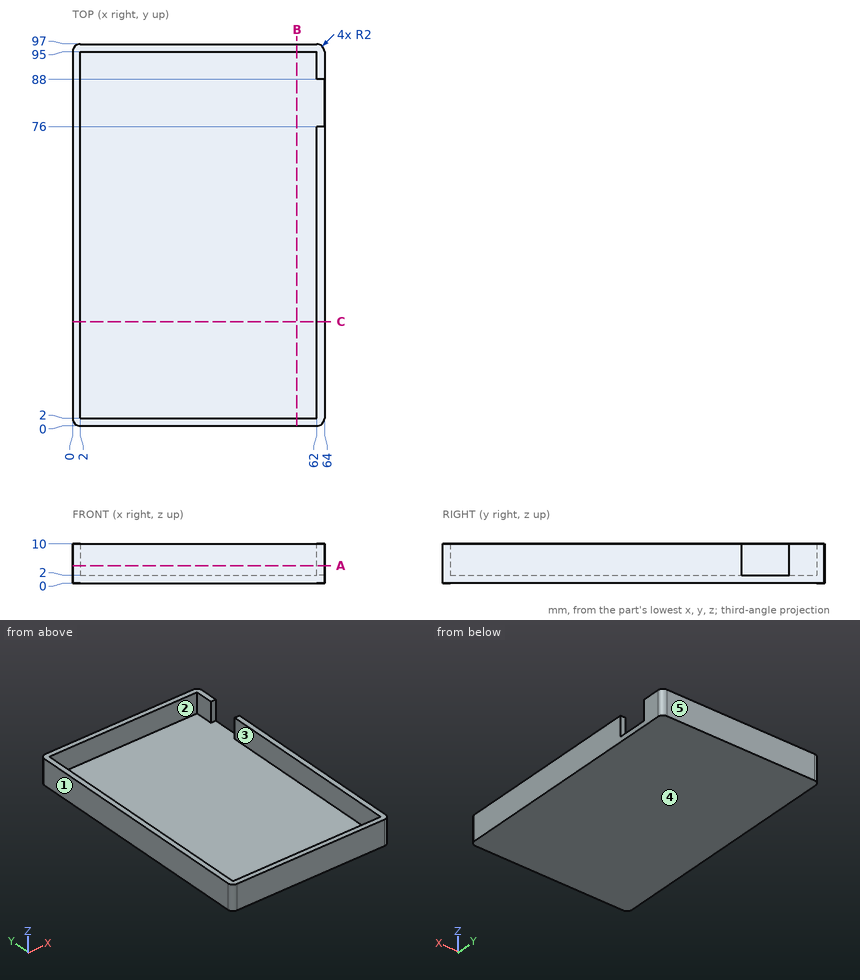
Input: dimensioned drawing with shaded views. Units: mm. Origin: part minimum x, y, z. A direction names the side the tool comes from. Give positions to 0.01 mm unless a question says otherwise; leave off trailing zeros. Order: outer loops, then holes, each group sorted by start corner. A loop starts at its lowest first (then second) coordinate and runs counter-clockwise, first axis right, second up. Notation, with made-up numbers: (56, 55) -> (78, 55) arc R16 cw to (78, 65) -> close; hole circle Ø6 at (42.5, 61). An arc over 180 degrees is marked (long way). Answer as a JSON object with one key per item and string values.
Q1. Draft query along Y for the marked faces 3, 4 and 5. Return one class per face: released by +Y, released by -Y, zero draft, split by the parting line, or undercut.
Entries:
{"face 3": "undercut", "face 4": "zero draft", "face 5": "released by +Y"}
Q2. Access query for the marked faces 1 and 2. Directions: +Z, -Z, +X, -X, +Y, -Y. A direction counts if a zero-diameter tool reaches every point of the face in a straight line with its end or side. Return the directions, or none.
Entries:
{"face 1": "+Z, -Z, -X, +Y, -Y", "face 2": "+Z"}
Q3. Section B-B (x = 57). Output: boundary loops of the cut face in (y, z), plus the area to 3 significant figures.
Entries:
{"outline": "(0, 0) -> (97, 0) -> (97, 10) -> (95, 10) -> (95, 2) -> (2, 2) -> (2, 10) -> (0, 10) -> close", "area": "226 mm^2"}
Q4. Section A-A (z = 4.5). Output: boundary loops of the cut face in (x, y), plus the area to 3 significant figures.
Entries:
{"outline": "(0, 2) arc R2 ccw to (2, 0) -> (62, 0) arc R2 ccw to (64, 2) -> (64, 76) -> (62, 76) -> (62, 2) -> (2, 2) -> (2, 95) -> (62, 95) -> (62, 88) -> (64, 88) -> (64, 95) arc R2 ccw to (62, 97) -> (2, 97) arc R2 ccw to (0, 95) -> close", "area": "601 mm^2"}
Q5. Material intervals for probe 1 along Y at (x, z) = (25, 7.25); probe 2 along X at (y, z) = (62, 8); probe 3 along Z at (x, y) = (61.5, 25), sorted ascending.
Entries:
{"probe 1": "y = 0 to 2, 95 to 97", "probe 2": "x = 0 to 2, 62 to 64", "probe 3": "z = 0 to 2"}
Q6. Section C-C (y = 26.5). Output: boundary loops of the cut face in (x, z).
Entries:
{"outline": "(0, 0) -> (64, 0) -> (64, 10) -> (62, 10) -> (62, 2) -> (2, 2) -> (2, 10) -> (0, 10) -> close"}
Q7. First-contact query: pin 1 (2.5 mm diameter, centred on x = 36.5, z = 4, fed in from -Y); pin 2 (1.6 mm diameter, centred on x = 63, z = 5, fed in from +Y). Flat tips, straight axial feed; report the tip coordinate or a pass-through.
Entries:
{"pin 1": "stops at y = 0", "pin 2": "stops at y = 96.99"}
